Design review of the part built by this model. Coordinates are the model's own, in mm. Face numbers are marked on the shaded views. A direction names the side the tool comes from. Give positions to 0.01 mm unless a question says otherwise; leave off trailing zeros. Write each loop counter-clockwise with the first axis right and the second up, starting at its lowest first coordinate (ties: lowest second). Pieces come first, ordered by that corner, then holes. Notation, with made-up numbers: M -33,43.25 L 21,43.25 A9 cw 21,60.25 Z; hole C 47,9.25 d3. An arc over 180 degrees is marked long. Write each question's results on one line, items separated by ' | '. Start each with the question number.
Autodesk Inventor part; units mm, degrees
ref_plane "YZ Plane" through (0, 0, 0) normal (1, 0, 0) x (0, 1, 0)
ref_plane "XZ Plane" through (0, 0, 0) normal (0, 1, 0) x (-1, 0, 0)
ref_plane "XY Plane" through (0, 0, 0) normal (0, 0, 1) x (1, 0, 0)
sketch "Sketch1" plane through (0, 0, 0) normal (0, 0, 1) x (1, 0, 0)
  line L0 (0, 0) -> (25.4, 0)
  line L1 (25.4, 0) -> (25.4, 133.35)
  line L2 (25.4, 133.35) -> (0, 133.35)
  line L3 (0, 133.35) -> (0, 0)
  line L4 (25.4, 0) -> (0, 0)
  line L5 (0, 0) -> (0, 92.075)
  line L6 (0, 92.075) -> (25.4, 92.075)
  line L7 (25.4, 92.075) -> (25.4, 0)
  line L8 (12.7, 0) -> (12.7, 85.725)
  line L9 (12.7, 0) -> (98.425, 0) construction
  circle A0 centre (12.7, 85.725) radius 3.175
  line L10 (12.7, 85.725) -> (12.7, 34.925)
  circle A1 centre (12.7, 34.925) radius 3.175
  dimension "d0" = 25.4
  dimension "d1" = 133.35
  dimension "d2" = 25.4
  dimension "d3" = 92.075
  dimension "d4" = 85.725
  dimension "d5" = 90
  dimension "d6" = 6.35
  dimension "d7" = 50.8
  dimension "d8" = 6.35
extrude "Extrusion1" add sketch "Sketch1" along normal blind 25.4
sketch "Sketch2" plane through (0, 133.35, 0) normal (0, 1, 0) x (1, 0, 0)
  line L0 (22.225, -22.225) -> (3.175, -22.225)
  line L1 (3.175, -22.225) -> (3.175, -3.175)
  line L2 (3.175, -3.175) -> (22.225, -3.175)
  line L3 (22.225, -3.175) -> (22.225, -22.225)
  dimension "d11" = 19.05
  dimension "d12" = 19.05
extrude "Extrusion2" cut sketch "Sketch2" against normal blind 254
sketch "Sketch3" plane through (25.4, 0, 0) normal (1, 0, 0) x (0, 0, -1)
  line L0 (0, 133.35) -> (-25.4, 133.35)
  line L1 (0, 0) -> (-25.4, 0)
  line L2 (-12.7, 133.35) -> (-12.7, 101.6)
  line L3 (-12.7, 133.35) -> (19.05, 133.35) construction
  circle A0 centre (-12.7, 101.6) radius 3.175
  dimension "d15" = 31.75
  dimension "d16" = 90
  dimension "d17" = 6.35
extrude "Extrusion3" cut sketch "Sketch3" against normal blind 254
sketch "Sketch4" plane through (0, 0, 25.4) normal (0, 0, 1) x (1, 0, 0)
  line L0 (25.4, 133.35) -> (0, 133.35)
  line L1 (0, 133.35) -> (0, 0)
  line L2 (12.7, 133.35) -> (12.7, 120.65)
  line L3 (12.7, 133.35) -> (25.4, 133.35) construction
  circle A0 centre (12.7, 120.65) radius 3.175
  dimension "d20" = 12.7
  dimension "d21" = 90
  dimension "d22" = 6.35
extrude "Extrusion4" cut sketch "Sketch4" against normal blind 25.4
properties part number "CatchSupport"
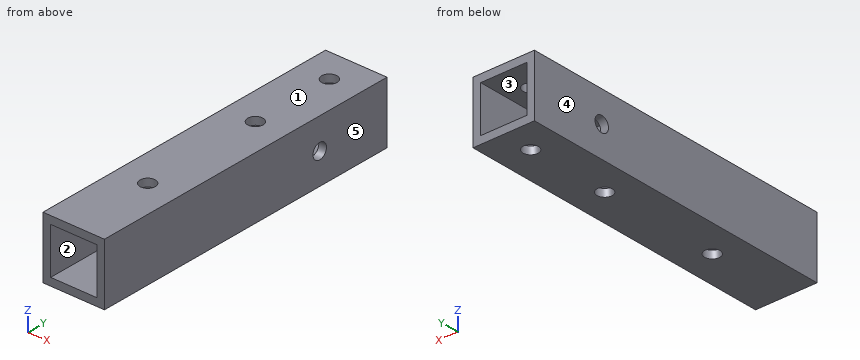
Q1. We need section A-A on x = 12.7. Count the separate pieces of the cut face and the enclosed holes in it, and give its area (3 significant figures).
Q2. Wall thickness on line 1 along Y through (x, z) = (12.7, 24.8) (3 decimals); line 2 along X through (y, z) = (8, 20) (3 decimals); line 3 along Z through (x, y) = (23.85, 101.6) (3 decimals): over which ranges is each line inside the solid? List them lowest first. Write a range as from..to.
Q3. For the marked faces 1 and 2, list the 3-axis set-ups (+Z, -Z, +X, -X, +Y, -Y) from which the entire face can be reached by the end or side of a thin tool; tool diameter is ignored.
Q4. We need section D-D on x = 6. Write out the cut boundary in (y, z) (3 decimals), and give its area (3 significant figures).
Q5. We need section B-B on z = 12.7. Write out the cut boundary in (x, y) (3 decimals), and give its area (3 significant figures).
Q6. We need section C-C on y = 120.65. Write out the cut boundary in (x, z) (3 decimals), and give its area (3 significant figures).
Q7. The part is to be moulded in two halves that separate along X. For the marked faces 3, 4 and 5, say which applies: pulls with the +X half, pulls with the -X half, needs draft (parallel to the pull), parting line crosses it, or undercut.
Answer sheet:
1) separate pieces: 8 | enclosed holes: 0 | area: 726 mm^2
2) line 1: 0..31.75, 38.1..82.55, 88.9..117.475, 123.825..133.35 | line 2: 0..3.175, 22.225..25.4 | line 3: 0..9.525, 15.875..25.4
3) face 1: +Z, +X, -X, +Y, -Y | face 2: +Y, -Y
4) outline: M 0,0 L 133.35,0 L 133.35,3.175 L 0,3.175 Z; M 0,22.225 L 133.35,22.225 L 133.35,25.4 L 0,25.4 Z | area: 847 mm^2
5) outline: M 0,0 L 3.175,0 L 3.175,98.425 L 0,98.425 Z; M 0,104.775 L 3.175,104.775 L 3.175,133.35 L 0,133.35 Z; M 22.225,0 L 25.4,0 L 25.4,98.425 L 22.225,98.425 Z; M 22.225,104.775 L 25.4,104.775 L 25.4,133.35 L 22.225,133.35 Z | area: 806 mm^2
6) outline: M 0,0 L 9.525,0 L 9.525,3.175 L 3.175,3.175 L 3.175,22.225 L 9.525,22.225 L 9.525,25.4 L 0,25.4 Z; M 15.875,0 L 25.4,0 L 25.4,25.4 L 15.875,25.4 L 15.875,22.225 L 22.225,22.225 L 22.225,3.175 L 15.875,3.175 Z | area: 242 mm^2
7) face 3: undercut | face 4: pulls with the -X half | face 5: pulls with the +X half
